```python
from build123d import *

# Parameters (mm, degrees)
F1_DEPTH = 75


with BuildPart() as f1:
    # F0 (on Front) → F1 (new body, symmetric)
    with BuildSketch(Plane.XZ):
        with BuildLine():
            Line((17.5, 7.844628), (17.5, 9.682458))
            ThreePointArc((17.5, 9.682458), (-20, 0), (17.5, -9.682458))
            Line((17.5, -9.682458), (17.5, -7.844628))
            Line((17.5, -7.844628), (22.5, -7.844628))
            Line((22.5, -7.844628), (22.5, 7.844628))
            Line((22.5, 7.844628), (17.5, 7.844628))
        make_face()
    extrude(amount=F1_DEPTH, both=True)


solid = f1.part
```
The model under review builds one solid part; all positions refer to its coordinate system, in mm. A direction names the side the tool comes from. Round coordinates to 2 decimals unless told otherwise and drop trailing zeros. Order: outer loops, then holes, each group sorted by start corner. A loop starts at its lowest first (then second) coordinate and runs counter-clockwise, first axis right, second up. Notation, with made-up numbers: (12, 64.25) -> (27, 64.25) arc R10 ccw to (27, 76.25) -> close; hole circle Ø1 at (-2, 67). An arc over 180 degrees is marked (long way). Use a Markdown table: item, result.
Q1. We need section B-B on x = -6. Write out the cut boundary in (y, z).
Values:
| item | result |
|---|---|
| outline | (-75, -19.08) -> (75, -19.08) -> (75, 19.08) -> (-75, 19.08) -> close |
Q2. We need section C-C on x = 4. Write out the cut boundary in (y, z), then the cut area to 3 significant figures.
Values:
| item | result |
|---|---|
| outline | (-75, -19.6) -> (75, -19.6) -> (75, 19.6) -> (-75, 19.6) -> close |
| area | 5,880 mm^2 |
Q3. Tool access review of faces 1 (the flat face through (20, -1, 7.845)), 2 (the flat face through (20, -1, -7.845)), 3 (the cylindrical face through (-19.986, -1.05, 0.738)): name each direction out of +Z, -Z, +X, -X, +Y, -Y from which nothing blocks a thin tool from reaching the whole face with its end or side.
Values:
| item | result |
|---|---|
| face 1 | +Z, +X, +Y, -Y |
| face 2 | -Z, +X, +Y, -Y |
| face 3 | +Y, -Y |
Q4. Clearance check with flat-ended pins moving along their axes: P1, Ø3, axis at x = -10.5, y = 8, coming from the -Z side; P2, Ø2, axis at y = 1, z = -9, coming from the +X side; P3, Ø10, axis at x = 6.5, y = -37, coming from the -Z side. State where each tip first meets the part, or that it passes through.
Values:
| item | result |
|---|---|
| P1 | stops at z = -17.86 |
| P2 | stops at x = 17.5 |
| P3 | stops at z = -19.94 |
Q5. We need section A-A on y = -57.5. Write out the cut boundary in (x, z), then the cut area to 3 significant figures.
Values:
| item | result |
|---|---|
| outline | (17.5, -9.68) -> (17.5, -7.84) -> (22.5, -7.84) -> (22.5, 7.84) -> (17.5, 7.84) -> (17.5, 9.68) arc R20 ccw (long way) to start |
| area | 1,300 mm^2 |
Q6. For line 1 (X direction, y = 36.5, z = -1); line 2 (Z direction, x = 18.5, y = -60.5); line 3 (X direction, y = 69, z = 17.5), list the stretches that pass through material, from the lowest coordinate up.
Values:
| item | result |
|---|---|
| line 1 | x = -19.97 to 22.5 |
| line 2 | z = -7.84 to 7.84 |
| line 3 | x = -9.68 to 9.68 |
